```python
from build123d import *

# Parameters (mm, degrees)
SKETCH1_R           = 12.25
BOSS_EXTRUDE1_DEPTH = 27
SKETCH2_R           = 11.414448149
BOSS_EXTRUDE2_DEPTH = 30
SKETCH3_R           = 2.5
BOSS_EXTRUDE3_DEPTH = 9.4
BOSS_EXTRUDE4_DEPTH = 1
SKETCH5_R           = 0.5
CUT_EXTRUDE1_DEPTH  = 2
SKETCH6_R           = 3.5
BOSS_EXTRUDE5_DEPTH = 1.5
SKETCH7_R           = 3.161406384
BOSS_EXTRUDE6_DEPTH = 1
FILLET1_R           = 1
CUT_EXTRUDE2_START  = -8
CUT_EXTRUDE2_DEPTH  = 8
SKETCH9_R           = 1.5
CUT_EXTRUDE3_DEPTH  = 6
SKETCH10_R          = 12.25
SKETCH10_R_2        = 11.97520775
CUT_EXTRUDE4_DEPTH  = 0.25
CUT_EXTRUDE7_START  = -0.5
SKETCH11_R          = 11.414448149
CUT_EXTRUDE7_DEPTH  = 0.5
FILLET2_R           = 0.5
SKETCH12_R          = 12.25
BOSS_EXTRUDE7_DEPTH = 0.25
SKETCH13_R          = 11.414448149
SKETCH13_R_2        = 11.154427358
CUT_EXTRUDE8_DEPTH  = 0.5
SKETCH3_2_R         = 2.5
BOSS_EXTRUDE8_DEPTH = 22.969653899


with BuildPart() as part:
    # Sketch1 → Boss-Extrude1 (new body)
    with BuildSketch(Plane.XY):
        Circle(SKETCH1_R)
    extrude(amount=-BOSS_EXTRUDE1_DEPTH)

    # Sketch2 → Boss-Extrude2 (add)
    with BuildSketch(Plane(origin=(0, 0, -27), x_dir=(-1, 0, 0), z_dir=(0, 0, -1))):
        Circle(SKETCH2_R)
    extrude(amount=BOSS_EXTRUDE2_DEPTH)

    # Sketch3 → Boss-Extrude3 (add)
    with BuildSketch(Plane.XY):
        Circle(SKETCH3_R)
    extrude(amount=BOSS_EXTRUDE3_DEPTH)

    # Sketch4 → Boss-Extrude4 (add, symmetric)
    with BuildSketch(Plane(origin=(0, 0, 0), x_dir=(0, 0, -1), z_dir=(1, 0, 0))):
        with BuildLine():
            Line((59.668792543, -7.131394742), (55.656453017, -7.131394742))
            ThreePointArc((55.656453017, -7.131394742), (54.525058274, -6), (55.656453017, -4.868605258))
            Line((55.656453017, -4.868605258), (59.668792543, -4.868605258))
            ThreePointArc((59.668792543, -4.868605258), (60.800187285, -6), (59.668792543, -7.131394742))
        make_face()
        with BuildLine():
            Line((59.668792543, 7.131394742), (55.656453017, 7.131394742))
            ThreePointArc((55.656453017, 7.131394742), (54.525058274, 6), (55.656453017, 4.868605258))
            Line((55.656453017, 4.868605258), (59.668792543, 4.868605258))
            ThreePointArc((59.668792543, 4.868605258), (60.800187285, 6), (59.668792543, 7.131394742))
        make_face()
    extrude(amount=BOSS_EXTRUDE4_DEPTH, both=True)

    # Sketch5 → Cut-Extrude1 (cut)
    with BuildSketch(Plane.ZY.offset(1)):
        with Locations((-59.668792543, -6)):
            Circle(SKETCH5_R)
        with Locations((-59.668792543, 6)):
            Circle(SKETCH5_R)
    extrude(amount=-CUT_EXTRUDE1_DEPTH, mode=Mode.SUBTRACT)

    # Sketch6 → Boss-Extrude5 (add)
    with BuildSketch(Plane.XY):
        Circle(SKETCH6_R)
    extrude(amount=BOSS_EXTRUDE5_DEPTH)

    # Sketch7 → Boss-Extrude6 (add)
    with BuildSketch(Plane(origin=(0, 0, -57), x_dir=(-1, 0, 0), z_dir=(0, 0, -1))):
        Circle(SKETCH7_R)
    extrude(amount=BOSS_EXTRUDE6_DEPTH)

    # Fillet1
    fillet1_edges = [part.edges().sort_by_distance(p)[0] for p in [
        (3.161406384, 0, -58),
    ]]
    fillet(fillet1_edges, radius=FILLET1_R - 0.0001)  # a hair under: the kernel refuses the full size

    # Sketch8 → Cut-Extrude2 (cut)
    with BuildSketch(Plane.XY.offset(9.4).offset(CUT_EXTRUDE2_START)):
        with BuildLine():
            Line((-1.842673821, 1.689542302), (1.842673821, 1.689542302))
            ThreePointArc((1.842673821, 1.689542302), (0, 2.5), (-1.842673821, 1.689542302))
        make_face()
    extrude(amount=CUT_EXTRUDE2_DEPTH, mode=Mode.SUBTRACT)

    # Sketch9 → Cut-Extrude3 (cut)
    with BuildSketch(Plane.XY):
        with Locations((-8.5, 0)):
            Circle(SKETCH9_R)
        with Locations((8.5, 0)):
            Circle(SKETCH9_R)
    extrude(amount=-CUT_EXTRUDE3_DEPTH, mode=Mode.SUBTRACT)

    # Sketch10 → Cut-Extrude4 (cut)
    with BuildSketch(Plane.XY.offset(-5)):
        Circle(SKETCH10_R)
        Circle(SKETCH10_R_2, mode=Mode.SUBTRACT)
    cut_extrude4 = extrude(amount=-CUT_EXTRUDE4_DEPTH, mode=Mode.SUBTRACT)

    # Mirror1: Cut-Extrude4 across plane
    add(cut_extrude4.mirror(Plane.XY.offset(-13.5)), mode=Mode.SUBTRACT)

    # Sketch11 → Cut-Extrude7 (cut)
    with BuildSketch(Plane(origin=(0, 0, -27.25), x_dir=(-1, 0, 0), z_dir=(0, 0, -1)).offset(CUT_EXTRUDE7_START)):
        Circle(SKETCH11_R)
    extrude(amount=CUT_EXTRUDE7_DEPTH, mode=Mode.SUBTRACT)


with BuildPart() as cut_extrude7_piece_1:
    # of the separate pieces the step leaves, piece 1, a body of its own (cut_extrude7_pieces)
    add(part.part.solids().sort_by_distance((12.25, 0, -27))[0])



with BuildPart() as cut_extrude7_piece_2:
    # of the separate pieces the step leaves, piece 2, a body of its own (cut_extrude7_pieces)
    add(part.part.solids().sort_by_distance((-3.161406384, 0, -57.0001))[0])

    # Fillet2
    fillet2_edges = [cut_extrude7_piece_2.edges().sort_by_distance(p)[0] for p in [
        (11.414448149, 0, -27.25),
    ]]
    fillet(fillet2_edges, radius=FILLET2_R)


with BuildPart() as cut_extrude7_piece_1_1:
    add(cut_extrude7_piece_1.part)

    add(cut_extrude7_piece_2.part)  # Boss-Extrude7 merges Cut-Extrude7 piece 2
    # Sketch12 → Boss-Extrude7 (add)
    with BuildSketch(Plane(origin=(0, 0, -27), x_dir=(-1, 0, 0), z_dir=(0, 0, -1))):
        with Locations(Location((0, 0, 0), (0, 0, 180))):
            Circle(SKETCH12_R)
    extrude(amount=BOSS_EXTRUDE7_DEPTH)

    # Sketch13 → Cut-Extrude8 (cut)
    with BuildSketch(Plane(origin=(0, 0, -54), x_dir=(-1, 0, 0), z_dir=(0, 0, -1))):
        Circle(SKETCH13_R)
        Circle(SKETCH13_R_2, mode=Mode.SUBTRACT)
    extrude(amount=-CUT_EXTRUDE8_DEPTH, mode=Mode.SUBTRACT)

    # Sketch3<2> → Boss-Extrude8 (add)
    with BuildSketch(Plane.XY):
        Circle(SKETCH3_2_R)
    extrude(amount=BOSS_EXTRUDE8_DEPTH)


solid = cut_extrude7_piece_1_1.part
```
CAD build for the part. Positions are in the model's coordinates, mm. A direction names the side the tool comes from. Round coordinates to 2 decimals unless told otherwise and drop trailing zeros. Order: outer loops, then holes, each group sorted by start corner. A loop starts at its lowest first (then second) coordinate and runs counter-clockwise, first axis right, second up.
Q1. Two-plate mould, pull along Y, no slides. Class faces 4 (the cylindrical face through (2.356, 0.836, 12.085)), 5 (the flat face through (1, -6, -59)), 6 (the cylindrical face through (7.3, -0.9, -3)): pulls with the +Y half, pulls with the -Y half, needs draft (parallel to the pull), parting line crosses it, or undercut.
Q2. Drop flat-ended pins along their axis: pin 1 (1 mm diameter, centred on x = 0, z = -58.5, fed in from -Y); pin 2 (3.5 mm diameter, centred on x = -0.5, y = 0, fed in from -Z); pin 3 (1.8 mm diameter, centred on y = 6.5, z = -58, fed in from +X). Give the stop position or say it passes through.
Q3. Slice it at B-B (x = 0). State how many separate pieces and enclosed holes the cut face has, and give its area (3 significant figures).
Q4. Wall check: L1, parallel to Z at x = 8, y = -2.25; L2, parallel to X at y = 10, z = -40; L3, parallel to Y at x = -5.5, z = -50.5. Give the ranges that are in metal, low to high.
Q5. Which spindle directions (+Z, -Z, +X, -X, +Y, -Y) get a long thin tool onto all of the face, cutting with end or side? Do faces 1 (the cylindrical face through (9.058, -6.946, -40.445)), 2 (the flat face through (-1, 6, -59)), 3 (the flat face through (0, 4.869, -58)). Say none if no direction does.
Q6. Slice it at C-C (z = -7). Write the cut outline in (x, y), and give its area (3 significant figures).
Q7. Slice it at A-A (z = 13). Write the cut outline in (x, y), and give its area (3 significant figures).
Results below:
1. face 4: parting line crosses it
1. face 5: needs draft
1. face 6: undercut
2. pin 1: stops at y = -7.13
2. pin 2: stops at z = -58
2. pin 3: stops at x = 1
3. separate pieces: 1
3. enclosed holes: 3
3. area: 1,480 mm2
4. L1: z = -57 to -27, -26.75 to 0
4. L2: x = -5.5 to 5.5
4. L3: y = -10 to 10
5. face 1: -Z
5. face 2: -Z, -X, +Y
5. face 3: -Z, +X, -X
6. outline: circle Ø24.5 at (0, 0)
6. area: 471 mm2
7. outline: circle Ø5 at (0, 0)
7. area: 19.6 mm2
